from build123d import *

# Parameters (mm, degrees)
F1_DEPTH = 5.25
F3_DEPTH = 5


# Not quite as in the source:
# - a feature names something its author has since deleted; it is built from what else it names


with BuildPart() as f1:
    # F0 (on Front) → F1 (new body, symmetric)
    with BuildSketch(Plane.XZ):
        with BuildLine():
            Line((-1, 0.25), (-1, 1.5))
            ThreePointArc((-1, 1.5), (-2.5, 0), (-1, -1.5))
            Line((-1, -1.5), (-1, -0.25))
            ThreePointArc((-1, -0.25), (-1.25, 0), (-1, 0.25))
        make_face()
        with BuildLine():
            ThreePointArc((0.5, 0), (0.0606601718, 1.0606601718), (-1, 1.5))
            Line((-1, 1.5), (-1, 0.25))
            ThreePointArc((-1, 0.25), (-0.8232233047, 0.1767766953), (-0.75, 0))
            ThreePointArc((-0.75, 0), (-0.8232233047, -0.1767766953), (-1, -0.25))
            Line((-1, -0.25), (-1, -1.5))
            ThreePointArc((-1, -1.5), (0.0606601718, -1.0606601718), (0.5, 0))
        make_face()
        with BuildLine():
            Line((1, 1.5), (-1, 1.5))
            ThreePointArc((-1, 1.5), (0.0606601718, 1.0606601718), (0.5, 0))
            ThreePointArc((0.5, 0), (0.0606601718, -1.0606601718), (-1, -1.5))
            Line((-1, -1.5), (1, -1.5))
            Line((1, -1.5), (1, 1.5))
        make_face()
    extrude(amount=F1_DEPTH, both=True)

    # F2 (on face) → F3 (cut, symmetric)
    with BuildSketch(Plane.XY.offset(1.5)):
        Polygon((-1, -4.9999998882), (0.5, -4.9999998882), (0.5, 4.9999998882), (-1, 4.9999998882), (-6.6263522021, 4.9999998882), (-6.6263522021, -4.9999998882), align=None)
    extrude(amount=F3_DEPTH, both=True, mode=Mode.SUBTRACT)


solid = f1.part
For this review, take the finished solid that the model builds, in its own axes (mm). A direction names the side the tool comes from. Coordinates: 2 decimals unless noted, no trailing zeros. Order: outer loops, then holes, each group sorted by start corner. A loop starts at its lowest first (then second) coordinate and runs counter-clockwise, first axis right, second up. Notation, with made-up numbers: (28.5, -10.5) -> (62.5, -10.5) arc R32 ccw to (62.5, 25.5) -> close; hole circle Ø3 at (86.25, 59.25). An arc over 180 degrees is marked (long way). Return JSON: item names as keys, results as strings.
1. We need section B-B on x = -2. Write out the cut boundary in (y, z), and give its area (3 significant figures).
Answer block:
{"outline": "(-5.25, -1.12) -> (-5, -1.12) -> (-5, 1.12) -> (-5.25, 1.12) -> close; (5, -1.12) -> (5.25, -1.12) -> (5.25, 1.12) -> (5, 1.12) -> close", "area": "1.12 mm²"}
2. The part is to be moulded in two halves that separate along Y. For faces 1 (the flat face through (1, 0, 0)), 2 (the flat face through (-0.6, 5, 0)), 3 (the flat face through (0, -5.25, 0)), say which applies: +Y half, -Y half, draft (parallel to the pull), parting line (faces both ways), or undercut.
Answer block:
{"face 1": "draft", "face 2": "undercut", "face 3": "-Y half"}
3. We need section C-C on y = -4.25. Write out the cut boundary in (x, z), and give its area (3 significant figures).
Answer block:
{"outline": "(0.5, -1.5) -> (1, -1.5) -> (1, 1.5) -> (0.5, 1.5) -> close", "area": "1.50 mm²"}
4. Machinability: for faces 4 (the flat face through (0.5, 0, 0)), 5 (the flat face through (0.7, 0, 1.5)), which of the approach directions +Z, -Z, +X, -X, +Y, -Y give a long, thin tool a straight path to every point of the face, cutting with its end or side? Answer none if there is none.
Answer block:
{"face 4": "+Z, -Z, -X", "face 5": "+Z, +X, -X, +Y, -Y"}
5. We need section A-A on x = 0.25. Write out the cut boundary in (y, z).
Answer block:
{"outline": "(-5.25, -1.5) -> (-5, -1.5) -> (-5, 1.5) -> (-5.25, 1.5) -> close; (5, -1.5) -> (5.25, -1.5) -> (5.25, 1.5) -> (5, 1.5) -> close"}
6. For pin 1 Ø0.9 at (y, z) = (-2, 0) entering from -X, flat-tipped, find the tip position at first contact; note if it passes through.
Answer block:
{"pin 1": "x = 0.5"}
7. For line 1 (Y direction, x = -0.9, z = -0.4); line 2 (X direction, y = 3.5, z = -0.8), list the stretches that pass through material, from the lowest coordinate up. Write a range as from..to.
Answer block:
{"line 1": "-5.25..-5, 5..5.25", "line 2": "0.5..1"}
